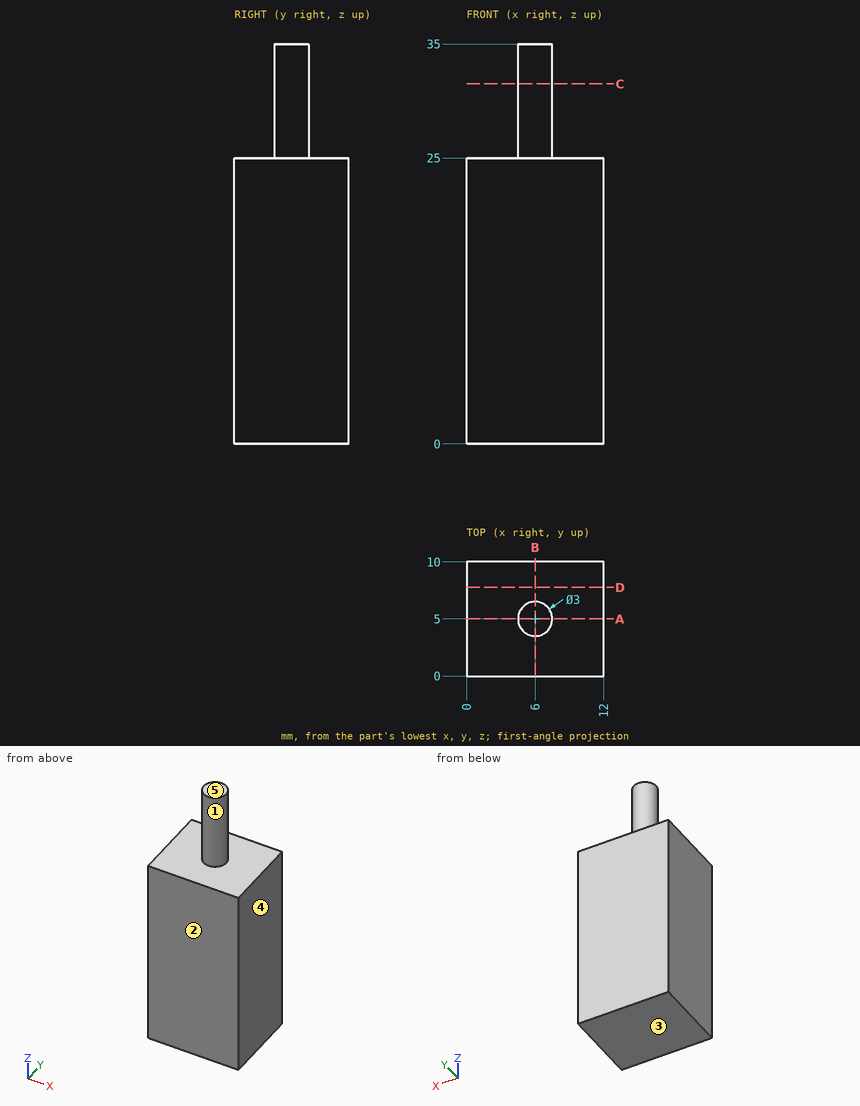
Answer from the drawing. Dimensions are ordinates in mm from the lowest x, y and z of the part. A direction names the side the tool comes from. Round coordinates to 2 decimals unless told otherwise and drop trailing zeros. Write each loop counter-clockwise with the first axis right and the second up, starting at its lowest first coordinate (ties: lowest second). Pieces come first, ordered by that corner, then holes. Notation, with made-up numbers: (18.25, 3) -> (58.25, 3) arc R17 cw to (58.25, 12) -> close; hole circle Ø8 at (-21, 7.25). An arc over 180 degrees is marked (long way). Answer in a Markdown table with one row per item. Add a question column.
1) Consider line 1 (Z direction, x = 5, y = 1); line 2 (Y direction, x = 7, z = 28); line 3 (X direction, y = 6.25, z = 30). Determine where each line is inside the solid, lowest interval first.
2) Given P1, Ø6, axis at x = 8.5, z = 27.5, coming from the +Y side, flat-ended and moving along its own axis, determine where the tip first touches the part or whether it passes through.
3) Which of the six approach directions +Z, -Z, +X, -X, +Y, -Y give full straight-line access (tool end or side, diameter ignored) to the marked faces 1 and 2?
4) Find section A-A, the plane y = 5. Determine the outline of the cut face in (x, z).
5) Find section B-B, the plane x = 6. Determine the outline of the cut face in (y, z), and give its area (3 significant figures).
6) Find section C-C, the plane z = 31.5. Determine the outline of the cut face in (x, y), and give its area (3 significant figures).
7) Determine the mould class of the marked faces 3, 4 and 5 for opening direction Z: pulls with the +Z half, pulls with the -Z half, needs draft (parallel to the pull), parting line crosses it, or undercut.
8) Find section D-D, the plane y = 7.75. Determine the outline of the cut face in (x, z).
Findings below:
| question | item | result |
|---|---|---|
| 1 | line 1 | 0 to 25 |
| 1 | line 2 | 3.88 to 6.12 |
| 1 | line 3 | 5.17 to 6.83 |
| 2 | P1 | y = 10 |
| 3 | face 1 | +Z |
| 3 | face 2 | +Z, -Z, +X, -X, -Y |
| 4 | outline | (0, 0) -> (12, 0) -> (12, 25) -> (7.5, 25) -> (7.5, 35) -> (4.5, 35) -> (4.5, 25) -> (0, 25) -> close |
| 5 | outline | (0, 0) -> (10, 0) -> (10, 25) -> (6.5, 25) -> (6.5, 35) -> (3.5, 35) -> (3.5, 25) -> (0, 25) -> close |
| 5 | area | 280 mm² |
| 6 | outline | circle Ø3 at (6, 5) |
| 6 | area | 7.07 mm² |
| 7 | face 3 | pulls with the -Z half |
| 7 | face 4 | needs draft |
| 7 | face 5 | pulls with the +Z half |
| 8 | outline | (0, 0) -> (12, 0) -> (12, 25) -> (0, 25) -> close |
